Can you work these out from the drawing? Everything is in mm from the part's minimum corner. A direction names the side the tool comes from. Round coordinates to 2 decimals unless told otherwise and drop trailing zeros. Loops run counter-clockwise (first coordinate to the right, second up) from the corner with the lowest first, then second, coordinate; pieces in that order, holes last. Notation, with made-up numbers: M -9,7 L 43,7 A30 ccw 43,37 Z; hole C -17,-29 d11. An arc over 180 degrees is marked long. Answer in a Markdown table with one row per item.
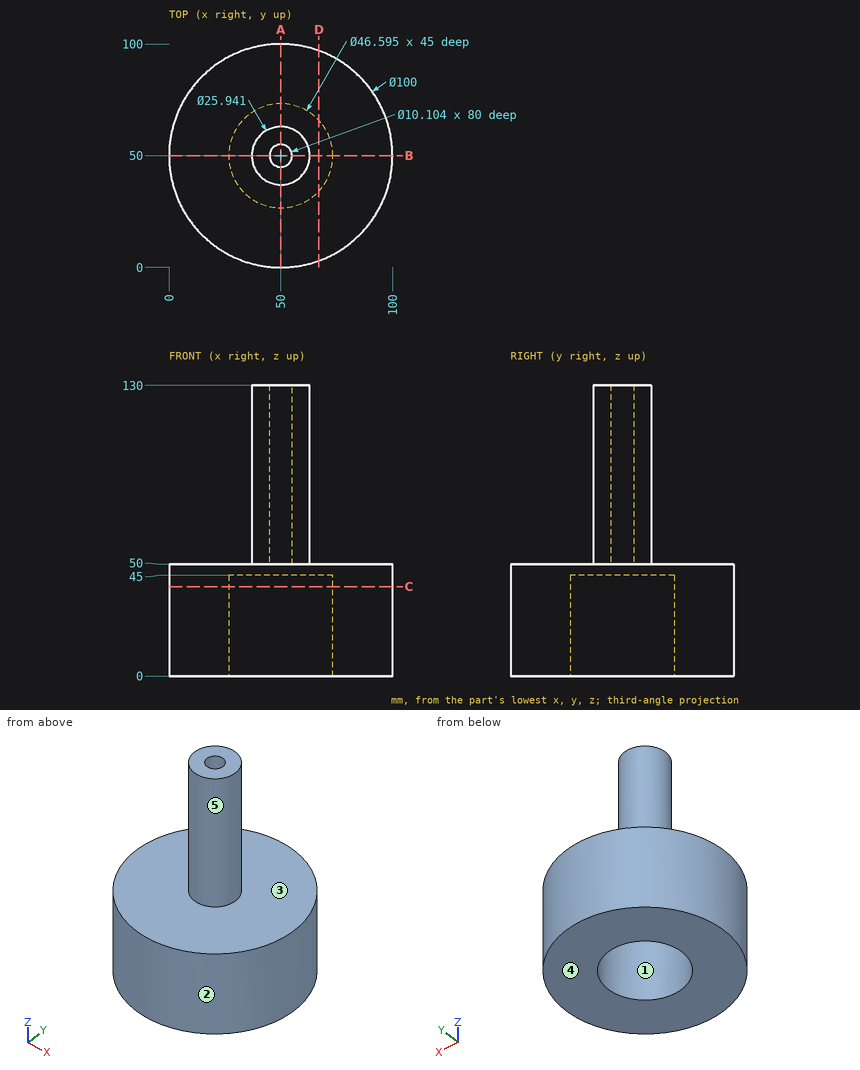
1) Which directions (+Z, -Z, +X, -X, +Y, -Y) give clear straight access to the entire face, cutting with the end or side of a thin tool? Please do the marked faces 4 and 5.
Computed:
| item | result |
|---|---|
| face 4 | -Z, +X, -X, +Y, -Y |
| face 5 | +Z |
2) I want a section at A-A, the plane x = 50. Please give me the cut outline in (y, z).
Computed:
| item | result |
|---|---|
| outline | M 0,0 L 26.7,0 L 26.7,45 L 73.3,45 L 73.3,0 L 100,0 L 100,50 L 62.97,50 L 62.97,130 L 55.05,130 L 55.05,50 L 44.95,50 L 44.95,130 L 37.03,130 L 37.03,50 L 0,50 Z |
3) I want a section at D-D, the plane x = 67. Please give me the cut outline in (y, z).
Computed:
| item | result |
|---|---|
| outline | M 2.98,0 L 34.07,0 L 34.07,45 L 65.93,45 L 65.93,0 L 97.02,0 L 97.02,50 L 2.98,50 Z |
4) If we mould it in two halves opening along X, with no side actions, what happens to the marked faces 1, 2 and 3? For each: released by +X, released by -X, zero draft, split by the parting line, or undercut.
Computed:
| item | result |
|---|---|
| face 1 | undercut |
| face 2 | split by the parting line |
| face 3 | zero draft |
5) Will these pins go through, and if not, where does the flat tip stop? P1, Ø12, axis at x = 30.5, y = 87, coming from the +Z side; P2, Ø12, axis at y = 61.5, z = 115, coming from the -X side.
Computed:
| item | result |
|---|---|
| P1 | stops at z = 50 |
| P2 | stops at x = 38.25 |
6) I want a section at C-C, the plane z = 40. Please give me the cut outline in (x, y) (1 decimal), plus the area to 3 significant figures.
Computed:
| item | result |
|---|---|
| outline | C 50,50 d100; hole C 50,50 d46.6 |
| area | 6,150 mm² |
7) I need wall thicknesses on line 1 (Y direction, x = 50, z = 13.5); line 2 (Y direction, x = 50, z = 86); line 3 (Z direction, x = 20, y = 49.5). Which ranges of each line are inside material? Lowest first, please.
Computed:
| item | result |
|---|---|
| line 1 | y = 0 to 26.7, 73.3 to 100 |
| line 2 | y = 37.03 to 44.95, 55.05 to 62.97 |
| line 3 | z = 0 to 50 |
